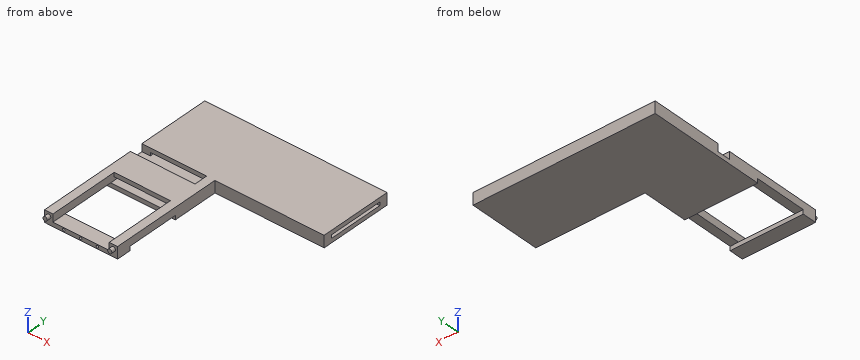
Autodesk Inventor part; units mm, degrees
ref_plane "Plano de trabajo4" through (-5.75, -5, -2.5) normal (1, 0, 0) x (0, 0, -1)
ref_plane "Plano de trabajo5" through (-27.5, -47.4, 0) normal (0, -1, 0) x (1, 0, 0)
ref_plane "YZ Plane" through (0, 0, 0) normal (1, 0, 0) x (0, 1, 0)
sketch "Boceto1" plane through (0, 0, 0) normal (0, 0, 1) x (1, 0, 0)
  line L0 (81, 20) -> (81, 63.5)
  line L1 (-27.5, 63.5) -> (-27.5, -5)
  line L2 (-27.5, -5) -> (16, -5)
  line L3 (16, -5) -> (16, 20)
  line L4 (11, 25) -> (11, -5)
  line L5 (-22.5, 58.5) -> (-22.5, -5)
  line L6 (11, 25) -> (81, 25)
  line L7 (-27.5, 63.5) -> (81, 63.5)
  line L8 (-22.5, 58.5) -> (81, 58.5)
  line L9 (16, 20) -> (81, 20)
  point P0 (0, 0)
  dimension "d7" = 5
  dimension "d68" = 5
  dimension "d69" = 33.5
  dimension "d74" = 5
  dimension "d75" = 33.5
  dimension "d76" = 5
  dimension "d77" = 70
  dimension "d111" = 30
extrude "Extrusión1" add sketch "Boceto1" against normal blind 2.5
extrude "Extrusión2" add sketch "Boceto1" along normal blind 1 contours L9 L3 L2 L4 L6 L0 | L8 L5 L2 L1 L7 L0
ref_plane "Plano de trabajo3" through (29.25, 58.5, 1) normal (0, 0, 1) x (1, 0, 0)
mirror "Simetría3" about plane through (29.25, 58.5, 1) normal (0, 0, 1) of "Extrusión2", "Extrusión1"
sketch "Boceto6" plane through (-27.5, 63.5, 4.5) normal (0, 0, 1) x (1, 0, 0)
  line L0 (108.5, -43.5) -> (43.5, -43.5)
  line L1 (0, -68.5) -> (0, 0)
  line L2 (0, -43.5) -> (0, -51.5)
  line L3 (43.5, -43.5) -> (43.5, -68.5)
  line L4 (0, -43.5) -> (38.5, -43.5)
  line L5 (38.5, -68.5) -> (38.5, -38.5)
  line L6 (0, -51.5) -> (38.5, -51.5)
  line L7 (38.5, -43.5) -> (38.5, -51.5)
  point P0 (27.5, -63.5)
  point P1 (43.5, -51.5)
  dimension "d78" = 8
extrude "Extrusión11" cut sketch "Boceto6" against normal blind 4.5
sketch "Boceto7" plane through (-27.5, -5, -2.5) normal (-1, 0, 0) x (0, 0, 1)
  line L0 (0, 0) -> (0, 68.5)
  line L1 (0, 0) -> (0, -42.4)
  line L2 (0, 0) -> (7, 0)
  line L3 (0, 0) -> (7, 0)
  line L4 (7, 0) -> (7, -42.4)
  line L5 (0, -42.4) -> (86.5, -192.2224)
  line L6 (86.5, -192.2224) -> (89, -192.2224)
  line L7 (89, -192.2224) -> (92.375, -190.2738)
  line L8 (2.5, 0) -> (2.5, -42.4)
  line L9 (0, 0) -> (7, 0)
  line L10 (0, 0) -> (2.5, 0)
  line L11 (86.5, -192.2224) -> (89, -192.2224)
  line L12 (89, -192.2224) -> (92.375, -190.2738)
  line L13 (2.5, -42.4) -> (89, -192.2224)
  line L14 (0, -42.4) -> (-1.0904, -42.4)
  line L15 (7, -42.4) -> (92.375, -190.2738)
  line L16 (86.5, -187.8923) -> (89.875, -185.9437)
  point P0 (2.5, 5)
  point P1 (4.5, 0)
  point P2 (-0.5452, -42.4)
  dimension "d81" = 42.4
  dimension "d82" = 173
  dimension "d88" = 120
  dimension "d108" = 5
ref_plane "Plano de trabajo4" through (-5.75, -5, -2.5) normal (1, 0, 0) x (0, 0, -1)
extrude "Extrusión12" add sketch "Boceto7" against normal blind 21.75 contours L2 L8 L13 L6 L5 L1
extrude "Extrusión13" add sketch "Boceto7" against normal blind 5 contours L2 L4 L15 L16 L13 L8
extrude "Extrusión14" add sketch "Boceto7" against normal blind 21.75 contours L13 L16 L15 L7
mirror "Simetría4" about plane through (-5.75, -5, -2.5) normal (1, 0, 0) of "Extrusión12", "Extrusión13", "Extrusión14"
sketch "Boceto8" plane through (-22.5, -47.4, 0) normal (0, 0.5, 0.866) x (1, 0, 0)
  line L0 (0, 0) -> (33.5, 0)
  line L1 (16.75, 0) -> (16.75, -5)
  circle A0 centre (16.75, -15.25) radius 10.25
  line L2 (16.75, -25.5) -> (16.75, -30.5)
  circle A1 centre (16.75, -41.5) radius 11
  line L3 (16.75, -52.5) -> (16.75, -57.5)
  circle A2 centre (16.75, -68.69) radius 11.19
  line L4 (16.75, -79.88) -> (16.75, -84.88)
  circle A3 centre (16.75, -96.38) radius 11.5
  line L5 (16.75, -107.88) -> (16.75, -112.88)
  circle A4 centre (16.75, -125.07) radius 12.19
  line L6 (16.75, -137.26) -> (16.75, -142.26)
  circle A5 centre (16.75, -155.01) radius 12.75
  point P0 (22.5, 41.0496)
  dimension "d105" = 25.5
  dimension "d94" = 5
  dimension "d95" = 20.5
  dimension "d96" = 5
  dimension "d97" = 5
  dimension "d98" = 5
  dimension "d99" = 5
  dimension "d100" = 5
  dimension "d101" = 22
  dimension "d102" = 22.38
  dimension "d103" = 23
  dimension "d104" = 24.38
extrude "Extrusión15" cut sketch "Boceto8" against normal blind 21.75
sketch "Boceto9" plane through (-27.5, 63.5, -2.5) normal (-1, 0, 0) x (0, 0, 1)
  line L0 (2.5, -51.5) -> (2.5, -110.9)
  line L1 (0, 0) -> (0, -110.9)
  line L2 (0, -110.9) -> (2.5, -110.9)
  line L3 (2.5, -110.9) -> (2.5, -70.9)
  line L4 (2.5, -70.9) -> (0, -70.9)
  line L5 (0, -70.9) -> (0, -110.9)
  line L6 (0, -43.5) -> (0, -110.9)
  line L7 (0, -102.4) -> (2.5, -102.4)
  point P0 (2.5, -63.5)
  point P1 (7, -110.9)
  dimension "d109" = 2.5
  dimension "d110" = 40
  dimension "d112" = 31.5
extrude "Extrusión16" cut sketch "Boceto9" against normal through all contours L0 L7 L1 L4
ref_plane "Plano de trabajo5" through (-27.5, -47.4, 0) normal (0, -1, 0) x (1, 0, 0)
sketch "Boceto10" plane through (-27.5, -47.4, 0) normal (0, -1, 0) x (1, 0, 0)
  line L0 (43.5, 0) -> (43.5, -2.5)
  line L1 (0, 86.5) -> (0, 89.875)
  line L2 (43.5, -2.5) -> (0, -2.5)
  line L3 (0, -2.5) -> (0, 89.875)
  line L4 (0, 89.875) -> (43.5, 89.875)
  line L5 (43.5, 89.875) -> (43.5, -2.5)
  point P0 (27.5, 0)
extrude "Extrusión17" cut sketch "Boceto10" along normal through all
sketch "Boceto11" plane through (-27.5, -47.4, 0) normal (0, -1, 0) x (1, 0, 0)
  line L0 (43.5, 4.5) -> (38.5, 4.5)
  line L1 (38.5, 0) -> (38.5, 4.5)
  line L2 (5, 0) -> (38.5, 0)
  line L3 (5, 4.5) -> (5, 0)
  line L4 (0, 4.5) -> (5, 4.5)
  line L5 (0, -2.5) -> (0, 4.5)
  line L6 (0, -2.5) -> (43.5, -2.5)
  line L7 (43.5, 4.5) -> (43.5, -2.5)
  line L8 (0, 0) -> (0, -2.5)
  line L9 (0, -1.25) -> (43.5, -1.25)
  line L10 (43.5, -2.5) -> (43.5, 4.5)
  circle A0 centre (2.5, 2) radius 1.25
  line L11 (108.5, 2) -> (5, 2)
  circle A1 centre (41, 2) radius 1.25
  circle A2 centre (11.5, -1.25) radius 0.75
  circle A3 centre (21.5, -1.25) radius 0.75
  circle A4 centre (31.5, -1.25) radius 0.75
  point P0 (27.5, 0)
  dimension "d117" = 2.5
  dimension "d118" = 2.5
  dimension "d119" = 38.5
  dimension "d120" = 1.5
  dimension "d121" = 1.5
  dimension "d122" = 1.5
  dimension "d123" = 10
  dimension "d124" = 10
  dimension "d125" = 12
extrude "Extrusión18" add sketch "Boceto11" along normal blind 2.5 contours A1 L11 | L11 A1 | A0
extrude "Extrusión19" cut sketch "Boceto11" against normal blind 2.5 contours A4 L9 | L9 A4 | A3 L9 | L9 A3 | A2 L9 | L9 A2
equation "\"d105\" = UnSol"
equation "\"d94\" = razon"
equation "\"d95\" = diezcen"
equation "\"d96\" = razon"
equation "\"d97\" = razon"
equation "\"d98\" = razon"
equation "\"d99\" = razon"
equation "\"d100\" = razon"
equation "\"d101\" = cincuentacen"
equation "\"d102\" = dossol"
equation "\"d103\" = veintecen"
equation "\"d104\" = cincosol"
equation "\"UnSol\" = 25.5"
equation "\"diezcen\" = 20.5"
equation "\"veintecen\" = 23"
equation "\"cincuentacen\" = 22"
equation "\"dossol\" = 22.38"
equation "\"cincosol\" = 24.38"
equation "\"razon\" = 5"
properties part number "V1"
The model under review builds one solid part; all positions refer to its coordinate system, in mm. Round coordinates to 2 decimals unless told otherwise and drop trailing zeros. Loops run counter-clockwise (first coordinate to the right, second up) from the corner with the lowest first, then second, coordinate; pieces in that order, holes last. Notation, with made-up numbers: (-11, 36) -> (40, 36) arc R23 cw to (40, 52) -> close; hole circle Ø1 at (59.25, 57.5). An arc over 180 degrees is marked (long way). Answer in a Markdown table with one row per item.
1) Consider section A-A, the plane y = -25.5. Write out the cut boundary in (x, z), plus the area to 3 significant figures.
Taken from the geometry:
| item | result |
|---|---|
| outline | (-27.5, 0) -> (-22.5, 0) -> (-22.5, 4.5) -> (-27.5, 4.5) -> close; (11, 0) -> (16, 0) -> (16, 4.5) -> (11, 4.5) -> close |
| area | 45.0 mm² |
2) Wall thickness on line 1 along X through (y, z) = (-45.55, -1.25); line 2 along Z through (x, y) = (25, 26.5); line 3 along Z through (x, y) = (-16, -45): over which ranges is each line inside the solid? List them lowest first.
Taken from the geometry:
| item | result |
|---|---|
| line 1 | x = -27.5 to -16.75, -15.25 to -6.75, -5.25 to 3.25, 4.75 to 16 |
| line 2 | z = -2.5 to 0, 2 to 4.5 |
| line 3 | z = -2.5 to -2, -0.5 to 0 |
3) Consider section B-B, the plane x = 49. Write out the cut boundary in (y, z), plus the area to 4 significant figures.
Taken from the geometry:
| item | result |
|---|---|
| outline | (20, -2.5) -> (63.5, -2.5) -> (63.5, 4.5) -> (20, 4.5) -> close; hole (25, 0) -> (58.5, 0) -> (58.5, 2) -> (25, 2) -> close |
| area | 237.5 mm² |
4) Consider section C-C, the plane y = 10. Write out the cut boundary in (x, z).
Taken from the geometry:
| item | result |
|---|---|
| outline | (-27.5, -2.5) -> (16, -2.5) -> (16, 4.5) -> (-27.5, 4.5) -> close; hole (-22.5, 0) -> (11, 0) -> (11, 2) -> (-22.5, 2) -> close |
5) For pin 1 Ø1 at (x, z) = (43, 1) entering from -Y; pin 2 Ø0.9 at (x, z) = (-16, -1.25) entering from -Y; pin 3 Ø1.6 at (x, z) = (-16, -1.5) entering from -Y; pin 4 Ø1 at (y, z) = (-14.5, -1.5) entering from +X, all flat-tipped, find the tip position at first contact; note any pin that passes through.
Taken from the geometry:
| item | result |
|---|---|
| pin 1 | stops at y = 20 |
| pin 2 | stops at y = -44.9 |
| pin 3 | stops at y = -47.4 |
| pin 4 | passes through |
